```python
from build123d import *

# Parameters (mm, degrees)
SKETCH1_W           = 11
SKETCH1_H           = 18
SKETCH1_W_2         = 5
SKETCH1_H_2         = 11
BOSS_EXTRUDE1_DEPTH = 4
BOSS_EXTRUDE2_DEPTH = 5
SKETCH3_R           = 0.5
CUT_EXTRUDE1_DEPTH  = 5
FILLET1_R           = 1
FILLET3_R           = 2
FILLET4_R           = 9
CUT_EXTRUDE2_DEPTH  = 10


with BuildPart() as part:
    # Sketch1 → Boss-Extrude1 (new body)
    with BuildSketch(Plane(origin=(0, 0, 0), x_dir=(1, 0, 0), z_dir=(0, 1, 0))):
        with Locations((-2.740875912, 16.357664234)):
            Rectangle(SKETCH1_W, SKETCH1_H)
        with Locations((-5.740875912, 30.857664234)):
            Rectangle(SKETCH1_W_2, SKETCH1_H_2)
    boss_extrude1 = extrude(amount=BOSS_EXTRUDE1_DEPTH)

    # Sketch2 → Boss-Extrude2 (add)
    with BuildSketch(Plane(origin=(-3.240875912, 0, 0), x_dir=(0, 0, -1), z_dir=(1, 0, 0))):
        with BuildLine():
            Line((34.537911903, 0), (25.357664234, 0))
            Line((25.357664234, 0), (25.357664234, -12.192130501))
            Line((25.357664234, -12.192130501), (34.537911903, -12.192130501))
            Line((34.537911903, -12.192130501), (34.537911903, -7.165523267))
            ThreePointArc((34.537911903, -7.165523267), (33.357664234, -5.7), (34.537911903, -4.234476733))
            Line((34.537911903, -4.234476733), (34.537911903, 0))
        make_face()
        with BuildLine():
            Line((36.357664234, 0), (34.537911903, 0))
            Line((34.537911903, 0), (34.537911903, -4.234476733))
            ThreePointArc((34.537911903, -4.234476733), (35.798507341, -4.531747353), (36.357664234, -5.7))
            ThreePointArc((36.357664234, -5.7), (35.798507341, -6.868252647), (34.537911903, -7.165523267))
            Line((34.537911903, -7.165523267), (34.537911903, -12.192130501))
            ThreePointArc((34.537911903, -12.192130501), (41.293121094, -6.613725887), (36.357664234, 0.62455532))
            Line((36.357664234, 0.62455532), (36.357664234, 0))
        make_face()
    boss_extrude2 = extrude(amount=-BOSS_EXTRUDE2_DEPTH)

    # Mirror1: Boss-Extrude1, Boss-Extrude2 across plane
    add(boss_extrude1.mirror(Plane(origin=(-8.240875912, 4, 0), x_dir=(0, 0, 1), z_dir=(1, 0, 0))))
    add(boss_extrude2.mirror(Plane(origin=(-8.240875912, 4, 0), x_dir=(0, 0, 1), z_dir=(1, 0, 0))))

    # Sketch3 → Cut-Extrude1 (cut)
    with BuildSketch(Plane(origin=(0, 4, 0), x_dir=(1, 0, 0), z_dir=(0, 1, 0))):
        with Locations(Location((-1.240875912, 20.357664234, 0), (0, 0, 270))):
            Circle(SKETCH3_R)
        with Locations(Location((-8.240875912, 12.357664234, 0), (0, 0, 270))):
            Circle(SKETCH3_R)
        with Locations(Location((-15.240875912, 20.357664234, 0), (0, 0, 270))):
            Circle(SKETCH3_R)
    extrude(amount=-CUT_EXTRUDE1_DEPTH, mode=Mode.SUBTRACT)

    # Fillet1
    fillet1_edges = [part.edges().sort_by_distance(p)[0] for p in [
        (-0.240875912, 4, -25.357664234),
        (-3.240875912, -4.234476733, -35.177416564),
        (-8.240875912, 4, -7.357664234),
        (-19.240875912, 4, -16.357664234),
        (-16.240875912, 4, -25.357664234),
        (2.759124088, 4, -16.357664234),
        (-13.240875912, -4.234476733, -35.177416564),
    ]]
    fillet(fillet1_edges, radius=FILLET1_R)

    # Fillet3
    fillet3_edges = [part.edges().sort_by_distance(p)[0] for p in [
        (-8.240875912, 0, -25.357664234),
    ]]
    fillet(fillet3_edges, radius=FILLET3_R)

    # Fillet4
    fillet4_edges = [part.edges().sort_by_distance(p)[0] for p in [
        (-8.240875912, -12.192130501, -25.357664234),
    ]]
    fillet(fillet4_edges, radius=FILLET4_R)

    # Sketch4 → Cut-Extrude2 (cut)
    with BuildSketch(Plane.ZY.offset(13.240875912)):
        Polygon((-36.357664234, 0.62455532), (-24.357664234, 4), (-36.357664234, 4), align=None)
    extrude(amount=-CUT_EXTRUDE2_DEPTH, mode=Mode.SUBTRACT)


solid = part.part
```
For this review, take the finished solid that the model builds, in its own axes (mm). A direction names the side the tool comes from. Give positions to 0.01 mm unless a question says otherwise; leave off trailing zeros. Loops run counter-clockwise (first coordinate to the right, second up) from the corner with the lowest first, then second, coordinate; pieces in that order, holes last. Notation, with made-up numbers: M -11.75,63.25 L 2.25,63.25 A20 ccw 2.25,86.25 Z; hole C 10,44.25 d11. An arc over 180 degrees is marked long. One line per item, written item: value. Start each with the question number.
Q1. Add section B-B (x = 1). Give the boundary of the cut face in (y, z), and give its area (3 significant figures).
Q2. Add section D-D (y = -9.25). Give the boundary of the cut face in (x, z).
Q3. Add section A-A (x = -9.25). Give the boundary of the cut face in (y, z), and give its area (3 significant figures).
Q4. Add section C-C (z = -10). Give the boundary of the cut face in (x, y).
Q5. Draft analysis for pull direction Z (two halves, no side actions). For faces 4 (the face through (-3.241, -4, -32)), 5 (the face through (-8.171, -9.486, -27.924)), 6 (the face through (-8.219, 2.028, -12.857)), state which applies: released by +Z, released by -Z, zero draft, split by the parting line, or undercut.
Q6. Machinability: for faces 1 (the face through (0, 1, -25.358)), 2 (the face through (-16.28, 3.7, -25.07)), 3 (the face through (-16, 1, -25.358)), which of the approach directions +Z, -Z, +X, -X, +Y, -Y give a long, thin tool a straight path to every point of the face, cutting with its end or side? Answer none if there is none.
Q7. For L1, parallel to Y at x = 0.25, z = -24; L2, parallel to X at y = -7, z = -27; L3, parallel to Z at x = -1.5, y = 1, list the stretches that pass through material, from the lowest coordinate up.
Q8. Clearance check with flat-ended pins moving along their axes: pin 1 Ø2.5 at (x, y) = (-15, 2) entering from -Z; pin 2 Ø9 at (x, z) = (-5, -12.5) entering from -Y; pin 3 Ø1.3 at (x, y) = (-8.5, -2.5) entering from +Z. State where each tip first meets the part, or that it passes through.
Reply:
1. outline: M 0,-25.36 L 3,-25.36 A1 ccw 4,-24.36 L 4,-8.36 A1 ccw 3,-7.36 L 0,-7.36 Z
1. area: 71.6 mm²
2. outline: M -13.24,-40.3 L -3.24,-40.3 L -3.24,-27.7 L -13.24,-27.7 Z
3. outline: M -12.19,-34.54 A6.5 ccw 0.62,-36.36 L 4,-24.36 L 4,-8.36 A1 ccw 3,-7.36 L 0,-7.36 L 0,-23.36 A2 cw -2,-25.36 L -3.19,-25.36 A9 ccw -12.19,-34.36 Z; hole C -5.7,-34.86 d3
3. area: 253 mm²
4. outline: M -19.24,0 L 2.76,0 L 2.76,3 A1 ccw 1.76,4 L -18.24,4 A1 ccw -19.24,3 Z
5. face 4: zero draft
5. face 5: released by +Z
5. face 6: undercut
6. face 1: -Z, +X, +Y, -Y
6. face 2: -Z, -X, +Y
6. face 3: -Z, -X, +Y, -Y
7. L1: 0 to 4
7. L2: -13.24 to -3.24
7. L3: -25.36 to -20.79, -19.93 to -7.36
8. pin 1: z = -25.36
8. pin 2: y = 0
8. pin 3: z = -25.35
